Build history of the part. All positions in model axes, mm. Face numbers are marked on the shaded views. A direction names the side the tool comes from. Round coordinates to 2 decimals unless told otherwise and drop trailing zeros. Write each loop counter-clockwise with the first axis right and the second up, starting at its lowest first coordinate (ties: lowest second). Pieces come first, ordered by that corner, then holes. Notation, with made-up numbers: (52.25, 58) -> (108.25, 58) arc R10 ccw to (108.25, 62) -> close; hole circle Ø3 at (-28.75, -9.75). An arc over 180 degrees is marked (long way). Return JSON: item names as keys, results as strings.
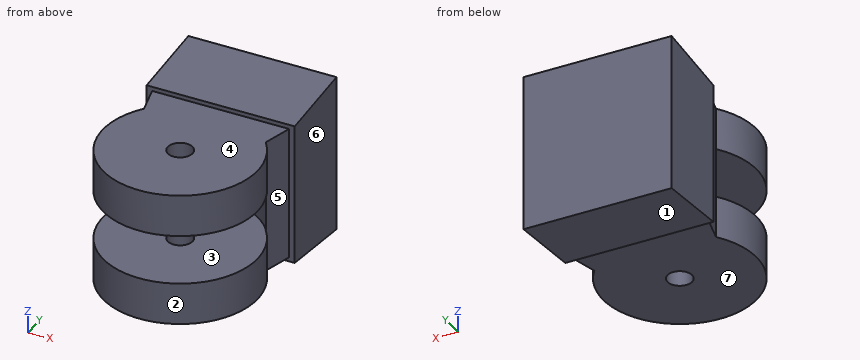
from build123d import *

# Parameters (mm, degrees)
SALIENTE_EXTRUIR1_DEPTH = 38.1
SALIENTE_EXTRUIR2_DEPTH = 34.29
CROQUIS3_R              = 39.658757808
CORTAR_EXTRUIR1_DEPTH   = 12.7
CROQUIS4_R              = 6.35
CORTAR_EXTRUIR2_DEPTH   = 131.416915542


with BuildPart() as part:
    # Croquis1 → Saliente-Extruir1 (new, symmetric)
    with BuildSketch(Plane(origin=(0, 0, 0), x_dir=(0, 0, -1), z_dir=(1, 0, 0))):
        Polygon((-40.64, 20.319999995), (-36.486122257, -20.319999995), (0, -20.319999995), (36.486122257, -20.319999995), (40.64, 20.319999995), align=None)
    extrude(amount=SALIENTE_EXTRUIR1_DEPTH, both=True)

    # Croquis2 → Saliente-Extruir2 (add, symmetric)
    with BuildSketch(Plane.XY):
        with BuildLine():
            Line((35.223664747, -20.319999995), (31.209635447, -35.506729715))
            ThreePointArc((31.209635447, -35.506729715), (0.114127167, -99.172386969), (-31.348920302, -35.687560492))
            Line((-31.348920302, -35.687560492), (-35.223664747, -20.319999995))
            Line((-35.223664747, -20.319999995), (35.223664747, -20.319999995))
        make_face()
    extrude(amount=SALIENTE_EXTRUIR2_DEPTH, both=True)

    # Croquis3 → Cortar-Extruir1 (cut, symmetric)
    with BuildSketch(Plane.XY):
        with Locations((0, -59.689999995)):
            Circle(CROQUIS3_R)
    extrude(amount=CORTAR_EXTRUIR1_DEPTH, both=True, mode=Mode.SUBTRACT)

    # Croquis4 → Cortar-Extruir2 (cut, through all)
    with BuildSketch(Plane.XY.offset(34.29)):
        with Locations((0, -59.689999995)):
            Circle(CROQUIS4_R)
    extrude(amount=-CORTAR_EXTRUIR2_DEPTH, mode=Mode.SUBTRACT)


solid = part.part
Q1. Saw through at D-D on y = -39.5. List the corners of the cut face in (x, z), then the cut area to 3 significant figures.
Verdict:
{"outline": "(-33.93, -34.29) -> (33.93, -34.29) -> (33.93, -12.7) -> (-33.93, -12.7) -> close; (-33.93, 12.7) -> (33.93, 12.7) -> (33.93, 34.29) -> (-33.93, 34.29) -> close", "area": "2,930 mm²"}
Q2. Saw through at A-A on y = -59.69. List the corners of the cut face in (x, z).
Verdict:
{"outline": "(-39.48, -34.29) -> (-6.35, -34.29) -> (-6.35, -12.7) -> (-39.48, -12.7) -> close; (-39.48, 12.7) -> (-6.35, 12.7) -> (-6.35, 34.29) -> (-39.48, 34.29) -> close; (6.35, -34.29) -> (39.48, -34.29) -> (39.48, -12.7) -> (6.35, -12.7) -> close; (6.35, 12.7) -> (39.48, 12.7) -> (39.48, 34.29) -> (6.35, 34.29) -> close"}
Q3. Saw through at B-B on x = 0. List the corners of the cut face in (y, z), then the cut area to 3 significant figures.
Verdict:
{"outline": "(-99.17, -34.29) -> (-66.04, -34.29) -> (-66.04, -12.7) -> (-99.17, -12.7) -> close; (-99.17, 12.7) -> (-66.04, 12.7) -> (-66.04, 34.29) -> (-99.17, 34.29) -> close; (-53.34, -34.29) -> (-20.32, -34.29) -> (-20.32, -36.49) -> (20.32, -40.64) -> (20.32, 40.64) -> (-20.32, 36.49) -> (-20.32, 34.29) -> (-53.34, 34.29) -> (-53.34, 12.7) -> (-20.03, 12.7) -> (-20.03, -12.7) -> (-53.34, -12.7) -> close", "area": "5,980 mm²"}
Q4. Wall check: L1, parallel to Z at x = 31, y = -42.5; L2, parallel to Y at x = 0, z = 22; L3, parallel to X at y = -11, z = 17. Give the ranges that are in metal, low to high.
Verdict:
{"L1": "z = -34.29 to -12.7, 12.7 to 34.29", "L2": "y = -99.17 to -66.04, -53.34 to 20.32", "L3": "x = -38.1 to 38.1"}
Q5. Saw through at C-C on z = -27. List the corners of the cut face in (x, y), then the cut area to 3 significant figures.
Verdict:
{"outline": "(-38.1, -20.32) -> (-35.22, -20.32) -> (-31.35, -35.69) arc R39.48 ccw (long way) to (31.21, -35.51) -> (35.22, -20.32) -> (38.1, -20.32) -> (38.1, 20.32) -> (-38.1, 20.32) -> close; hole circle Ø12.7 at (0, -59.69)", "area": "8,210 mm²"}
Q6. Pin check, flat tips, straight feed: pin 1 Ø10 at (x, y) = (-14, -85) entering from -Z; pin 2 Ø12 at (y, z) = (3.5, -2.5) entering from +X; pin 3 Ø20.5 at (x, y) = (0, -59.69) entering from +Z. Stop position of each tip, or through.
Verdict:
{"pin 1": "stops at z = -34.29", "pin 2": "stops at x = 38.1", "pin 3": "stops at z = 34.29"}
Q7. 3-axis set-ups, long thin cutter, end or side, ignore diameter. For the marked faces 4, 5, 6 and 7: which of +Z, -Z, +X, -X, +Y, -Y reach the whole face in a straight line?
Verdict:
{"face 4": "+Z, +X, -X, -Y", "face 5": "+Z, -Z, +X", "face 6": "+Z, -Z, +X, +Y", "face 7": "-Z, +X, -X, -Y"}
Q8. Two-plate mould, pull along Y, no slides. Class the marked faces 1, 2 and 3: +Y half, -Y half, draft (parallel to the pull), parting line (faces both ways), or undercut.
Verdict:
{"face 1": "-Y half", "face 2": "undercut", "face 3": "draft"}
